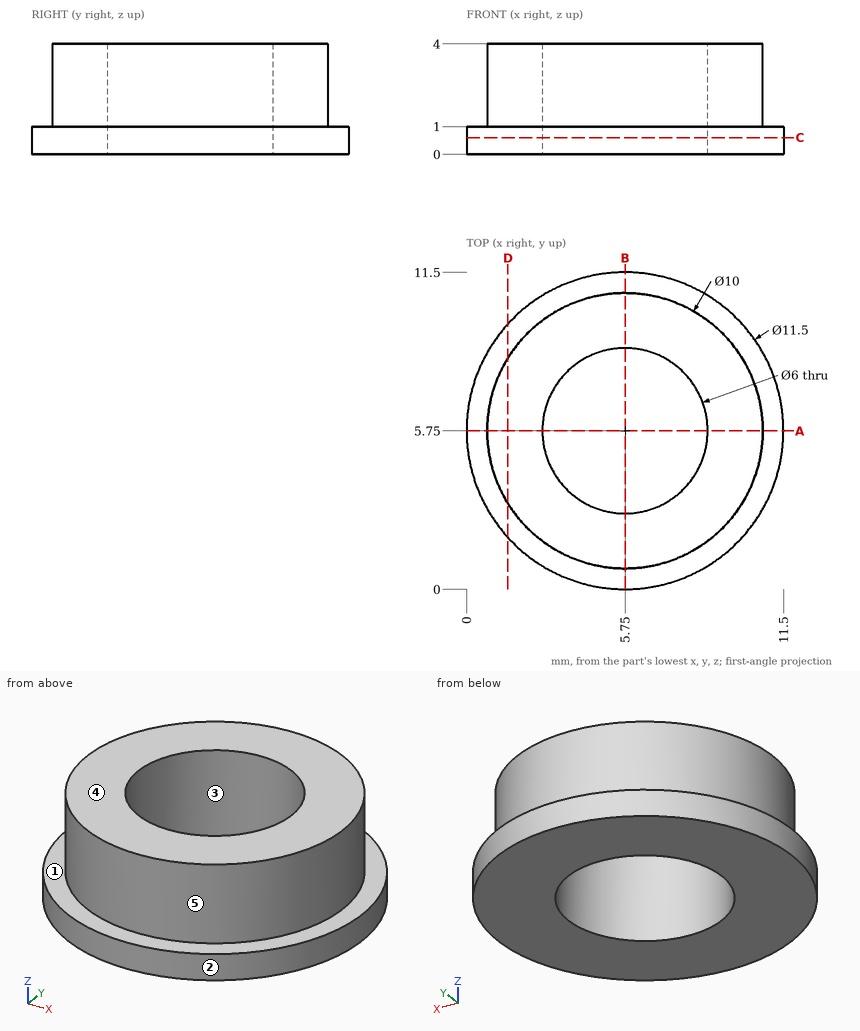
Design review of the part shown in the three views and the two pictorial views. Dimensions are in mm from the part's minimum x, y and z. A direction names the side the tool comes from. Give positions to 0.01 mm unless a question says otherwise; leave off trailing zeros. Write each loop counter-clockwise with the first axis right and the second up, starting at its lowest first coordinate (ties: lowest second). Pieces come first, ordered by that corner, then holes.
(1) Add section C-C (z = 0.6). Give the boundary of the cut face in (x, y).
Checked values:
outline: circle Ø11.5 at (5.75, 5.75); hole circle Ø6 at (5.75, 5.75)
(2) Clearance check with flat-ended pins moving along their axes: pin 1 Ø1.5 at (x, z) = (7, 0.5) entering from +Y; pin 2 Ø1 at (x, z) = (8, 3.5) entering from +Y. State where each tip first meets the part, or that it passes through.
Checked values:
pin 1: stops at y = 11.48
pin 2: stops at y = 10.43
(3) Tool access review of the marked faces 1 and 2: name each direction out of +Z, -Z, +X, -X, +Y, -Y from which nothing blocks a thin tool from reaching the whole face with its end or side.
Checked values:
face 1: +Z
face 2: +Z, -Z
(4) Mouldability with a two-part tool opening along X and no side actions: class the marked faces 3, 4 and 5 as +X half, -X half, draft (parallel to the pull), parting line (faces both ways), or undercut.
Checked values:
face 3: undercut
face 4: draft
face 5: parting line
(5) Add section D-D (x = 1.5). Give the boundary of the cut face in (y, z).
Checked values:
outline: (1.88, 0) - (9.62, 0) - (9.62, 1) - (8.38, 1) - (8.38, 4) - (3.12, 4) - (3.12, 1) - (1.88, 1) - close
(6) Wall thickness on line 1 along Y through (x, z) = (5.75, 2.9); line 2 along X through (y, z) = (5.5, 2.4); line 3 along X through (y, z) = (7.75, 2.5): over which ranges is each line inside the solid? List them lowest first.
Checked values:
line 1: y = 0.75 to 2.75, 8.75 to 10.75
line 2: x = 0.76 to 2.76, 8.74 to 10.74
line 3: x = 1.17 to 3.51, 7.99 to 10.33
(7) Add section A-A (y = 5.75). Give the boundary of the cut face in (x, z).
Checked values:
outline: (0, 0) - (2.75, 0) - (2.75, 4) - (0.75, 4) - (0.75, 1) - (0, 1) - close; (8.75, 0) - (11.5, 0) - (11.5, 1) - (10.75, 1) - (10.75, 4) - (8.75, 4) - close
